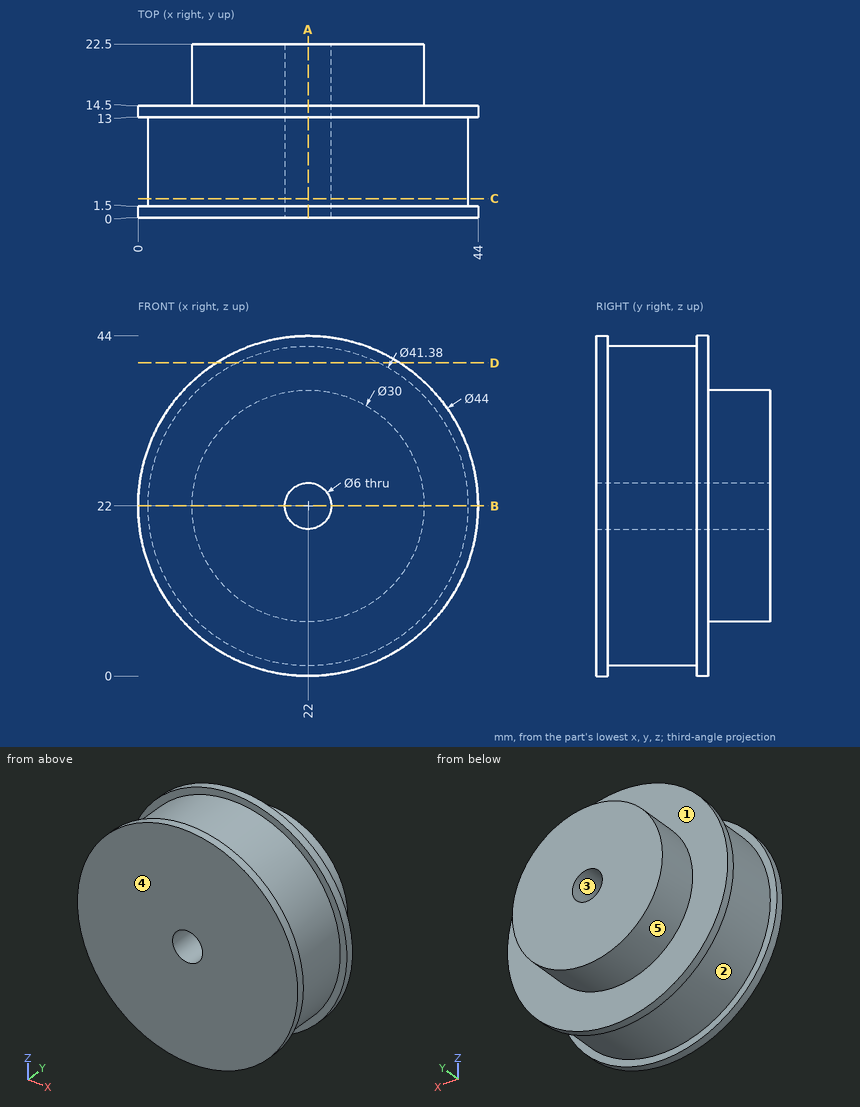
Part print with two shaded views. Sizes in mm from the minimum x, y, z corner. A direction names the side the tool comes from. Round coordinates to 2 decimals unless told otherwise and drop trailing zeros. Loops run counter-clockwise (first coordinate to the right, second up) from the corner with the lowest first, then second, coordinate; pieces in that order, holes last. Notation, with made-up numbers: (46.5, 11) - (105.5, 11) arc R19 cw to (105.5, 45) - close; hole circle Ø6 at (22, 35.5). An arc over 180 degrees is marked (long way). Answer as a JSON object with one key per item and string values.
Item 1: Pull direction Z, two halves, no side cores. Call the marked faces 1, 2 and 3: pulls with the +Z half, pulls with the -Z half, needs draft (parallel to the pull), parting line crosses it, or undercut.
Output:
{"face 1": "needs draft", "face 2": "parting line crosses it", "face 3": "undercut"}
Item 2: Band-saw the part on A-A on x = 22. List the corners of the cut face in (y, z), plus the area to 3 significant figures.
Output:
{"outline": "(0, 0) - (1.5, 0) - (1.5, 1.31) - (13, 1.31) - (13, 0) - (14.5, 0) - (14.5, 7) - (22.5, 7) - (22.5, 19) - (0, 19) - close; (0, 25) - (22.5, 25) - (22.5, 37) - (14.5, 37) - (14.5, 44) - (13, 44) - (13, 42.69) - (1.5, 42.69) - (1.5, 44) - (0, 44) - close", "area": "713 mm2"}
Item 3: Wall check: L1, parallel to Z at x = 22, y = 10.25; L2, parallel to Y at x = 8, z = 36; L3, parallel to Z at x = 22, y = 15.75. Give the ranges that are in metal, low to high.
Output:
{"L1": "1.31 to 19, 25 to 42.69", "L2": "0 to 14.5", "L3": "7 to 19, 25 to 37"}
Item 4: Pin check, flat tips, straight feed: pin 1 (1.5 mm diameter, centred on x = 9, z = 11.5, fed in from +Y); pin 2 (4 mm diameter, centred on x = 28, y = 11.5, fed in from +Z); pin 3 (4 mm diameter, centred on y = 11.5, z = 18, fed in from -X). Stop position of each tip, or through.
Output:
{"pin 1": "y = 14.5", "pin 2": "z = 43.5", "pin 3": "x = 0.16"}
Item 5: Band-saw the part on B-B on z = 22. List the corners of the cut face in (x, y), plus the area to 3 significant figures.
Output:
{"outline": "(0, 0) - (19, 0) - (19, 22.5) - (7, 22.5) - (7, 14.5) - (0, 14.5) - (0, 13) - (1.31, 13) - (1.31, 1.5) - (0, 1.5) - close; (25, 0) - (44, 0) - (44, 1.5) - (42.69, 1.5) - (42.69, 13) - (44, 13) - (44, 14.5) - (37, 14.5) - (37, 22.5) - (25, 22.5) - close", "area": "713 mm2"}
Item 6: Band-saw the part on C-C on y = 2.5. List the corners of the cut face in (x, z).
Output:
{"outline": "circle Ø41.38 at (22, 22); hole circle Ø6 at (22, 22)"}
Item 7: Band-saw the part on D-D on z = 40.5. List the corners of the cut face in (x, y), plus the area to 3 significant figures.
Output:
{"outline": "(10.09, 0) - (33.91, 0) - (33.91, 1.5) - (31.26, 1.5) - (31.26, 13) - (33.91, 13) - (33.91, 14.5) - (10.09, 14.5) - (10.09, 13) - (12.74, 13) - (12.74, 1.5) - (10.09, 1.5) - close", "area": "285 mm2"}
Item 8: Tool access for the marked faces 4 and 5: list every direction of +Z, -Z, +X, -X, +Y, -Y with a clear straight run to the whole face (end or side of a thin tool).
Output:
{"face 4": "+Z, -Z, +X, -X, -Y", "face 5": "+Y"}
